For this review, take the finished solid that the model builds, in its own axes (mm). Coordinates: 2 decimals unless noted, no trailing zeros. Write each loop counter-clockwise with the first axis right and the second up, starting at its lowest first coordinate (ties: lowest second). Pieces come first, ordered by that corner, then holes. Notation, with made-up numbers: (72.5, 23.5) -> (116.5, 23.5) arc R26 ccw to (116.5, 45.5) -> close; hole circle Ø4 at (-27, 20.25). An arc over 180 degrees is marked (long way). Put each result on its own line as item: value. Start each with the question number.
Item 1: To check wall thickness, follow L1, parallel to X at y = 53.25, z = 62.5; L2, parallel to X at y = 52.25, z = 51; L3, parallel to Y at x = 37, z = 44. State the ranges of each line that lie inside material, in increasing order.
Item 2: Consider section A-A on y = 55.75. Give the boundary of the cut face in (x, z).
Item 3: The part is to be moulded in two halves that separate along X. For faces 1 (the flat face through (-0.2, 60.5, 140)), 2 (the flat face through (-40.197, 47.905, 74.09)), 3 (the cylindrical face through (-0.586, 59.997, 74.09)), say which applies: +X half, -X half, draft (parallel to the pull), parting line (faces both ways), or undercut.
Item 4: Consider section B-B on z = 84. Give the boundary of the cut face in (x, y), and give its area (3 significant figures).
Item 5: Consider section C-C on x = 1. Give the boundary of the cut face in (y, z).
Item 6: Insertion check: P1, Ø3, axis at x = -13.5, z = 99.5, coming from the -Y side; P2, Ø3, axis at y = 50.5, z = 121.5, coming from the +X side; P3, Ø4, axis at x = 27, z = 42.5, coming from the -Y side. Each pin has a flat end and moves straight along its axis. Give the tip position at first contact, or say it passes through.
```python
from build123d import *

# Parameters (mm, degrees)
BOSS_EXTRUDE1_DEPTH = 10
BOSS_EXTRUDE2_DEPTH = 130
CUT_EXTRUDE1_DEPTH  = 130


with BuildPart() as part:
    # Sketch1 → Boss-Extrude1 (new, symmetric)
    with BuildSketch(Plane.XY):
        with BuildLine():
            Line((38.567256581, 45.962666587), (25.711504387, 30.641777725))
            ThreePointArc((25.711504387, 30.641777725), (0, 40), (-25.711504387, 30.641777725))
            Line((-25.711504387, 30.641777725), (-38.567256581, 45.962666587))
            ThreePointArc((-38.567256581, 45.962666587), (0, 60), (38.567256581, 45.962666587))
        make_face()
    extrude(amount=BOSS_EXTRUDE1_DEPTH, both=True)

    # Sketch4 → Cut-Extrude1 (cut)
    with BuildSketch(Plane.XY.offset(10)):
        with BuildLine():
            Line((-38.567256581, 45.962666587), (-25.711504387, 30.641777725))
            ThreePointArc((-25.711504387, 30.641777725), (0, 40), (25.711504387, 30.641777725))
            Line((25.711504387, 30.641777725), (38.567256581, 45.962666587))
            ThreePointArc((38.567256581, 45.962666587), (0, 60), (-38.567256581, 45.962666587))
        make_face()
    extrude(amount=-CUT_EXTRUDE1_DEPTH, mode=Mode.SUBTRACT)


with BuildPart() as body_2:
    # Sketch3 → Boss-Extrude2 (new body)
    with BuildSketch(Plane.XY.offset(10)):
        with BuildLine():
            Line((-41.78119463, 49.792888803), (-38.567256581, 45.962666587))
            ThreePointArc((-38.567256581, 45.962666587), (0, 60), (38.567256581, 45.962666587))
            Line((38.567256581, 45.962666587), (41.78119463, 49.792888803))
            ThreePointArc((41.78119463, 49.792888803), (0, 65), (-41.78119463, 49.792888803))
        make_face()
    extrude(amount=BOSS_EXTRUDE2_DEPTH)


solid = body_2.part
```
Return value:
1. L1: -37.28 to -27.65, 27.65 to 37.28
1. L2: -38.66 to -29.49, 29.49 to 38.66
1. L3: 47.23 to 53.44
2. outline: (-33.42, 10) -> (-22.18, 10) -> (-22.18, 140) -> (-33.42, 140) -> close; (22.18, 10) -> (33.42, 10) -> (33.42, 140) -> (22.18, 140) -> close
3. face 1: draft
3. face 2: -X half
3. face 3: undercut
4. outline: (-41.78, 49.79) -> (-38.57, 45.96) arc R60 cw to (38.57, 45.96) -> (41.78, 49.79) arc R65 ccw to start
4. area: 436 mm^2
5. outline: (59.99, 10) -> (64.99, 10) -> (64.99, 140) -> (59.99, 140) -> close
6. P1: y = 58.09
6. P2: x = 41.78
6. P3: y = 52.53
